Design review of the part built by this model. Coordinates are the model's own, in mm. A direction names the side the tool comes from. Give positions to 0.01 mm unless a question says otherwise; leave off trailing zeros. Loops run counter-clockwise (first coordinate to the right, second up) from the corner with the lowest first, then second, coordinate; pieces in that order, holes last. Notation, with made-up numbers: (63.5, -13.75) - (120.5, -13.75) arc R8 ccw to (120.5, -4.75) - close; hole circle Ø9 at (-26.75, 45.25). An arc over 180 degrees is marked (long way). Write each question's results on one line, items separated by ' | '.
```python
from build123d import *

# Parameters (mm, degrees)
F0_W     = 103.7199497223
F0_H     = 93.8791483641
F1_DEPTH = 83.4754128009
F5_DEPTH = 25.4


with BuildPart() as f1:
    # F0 (on Top) → F1 (new body)
    with BuildSketch(Plane.XY):
        with Locations((4.3902695179, -5.4262652993)):
            Rectangle(F0_W, F0_H)
    extrude(amount=F1_DEPTH)

    # F4 (on face) → F5 (join)
    with BuildSketch(Plane(origin=(41.7745485902, 0, 0), x_dir=(0, -1, 0), z_dir=(-1, 0, 0))):
        with BuildLine():
            ThreePointArc((33.5486456752, 83.4754128009), (25.6043620093, 102.6546101703), (6.4251646399, 110.5988938361))
            Line((6.4251646399, 110.5988938361), (6.4251646399, 83.4754128009))
            Line((6.4251646399, 83.4754128009), (33.5486456752, 83.4754128009))
        make_face()
        with BuildLine():
            Line((6.4251646399, 83.4754128009), (6.4251646399, 110.5988938361))
            ThreePointArc((6.4251646399, 110.5988938361), (-12.7540327294, 102.6546101703), (-20.6983163953, 83.4754128009))
            Line((-20.6983163953, 83.4754128009), (6.4251646399, 83.4754128009))
        make_face()
    extrude(amount=F5_DEPTH)


solid = f1.part
```
Item 1: We need section A-A on y = -9. Give the boundary of the cut face in (x, z).
Output values:
outline: (-47.47, 0) - (56.25, 0) - (56.25, 83.48) - (41.77, 83.48) - (41.77, 110.48) - (16.37, 110.48) - (16.37, 83.48) - (-47.47, 83.48) - close
Item 2: Tool access review of faces 1 (the face through (41.775, -6, 94)), 2 (the face through (4, -52.366, 41)), 3 (the face through (16.375, -6, 94)): name each direction out of +Z, -Z, +X, -X, +Y, -Y from which nothing blocks a thin tool from reaching the whole face with its end or side.
Output values:
face 1: +Z, +X, +Y, -Y | face 2: +Z, -Z, +X, -X, -Y | face 3: +Z, -X, +Y, -Y
Item 3: Wall thickness on probe 1 along Z at (x, y) = (43.5, -20.5); probe 2 along X at (y, z) = (-26, 90); probe 3 along Z at (x, y) = (30, -7): over which ranges is each line inside the solid? List them lowest first.
Output values:
probe 1: z = 0 to 83.48 | probe 2: x = 16.37 to 41.77 | probe 3: z = 0 to 110.59
Item 4: We need section D-D on y = -29. Give the boundary of the cut face in (x, z).
Output values:
outline: (-47.47, 0) - (56.25, 0) - (56.25, 83.48) - (41.77, 83.48) - (41.77, 98.51) - (16.37, 98.51) - (16.37, 83.48) - (-47.47, 83.48) - close
Item 5: We need section B-B on z = 102.5. Give the boundary of the cut face in (x, y), then the cut area to 3 significant figures.
Output values:
outline: (16.37, -25.76) - (41.77, -25.76) - (41.77, 12.91) - (16.37, 12.91) - close | area: 982 mm²
Item 6: Clearance check with flat-ended pins moving along their axes: P1, Ø8, axis at x = 24.5, y = 8.5, coming from the +Z side; P2, Ø1, axis at y = -16.5, z = 93.5, coming from the +X side; P3, Ø4, axis at x = 36, y = -29, coming from the +Z side. State where each tip first meets the part, or that it passes through.
Output values:
P1: stops at z = 108.3 | P2: stops at x = 41.77 | P3: stops at z = 101.15
Item 7: We need section C-C on x = -21. Give the boundary of the cut face in (y, z), then the cut area to 3 significant figures.
Output values:
outline: (-52.37, 0) - (41.51, 0) - (41.51, 83.48) - (-52.37, 83.48) - close | area: 7,840 mm²
